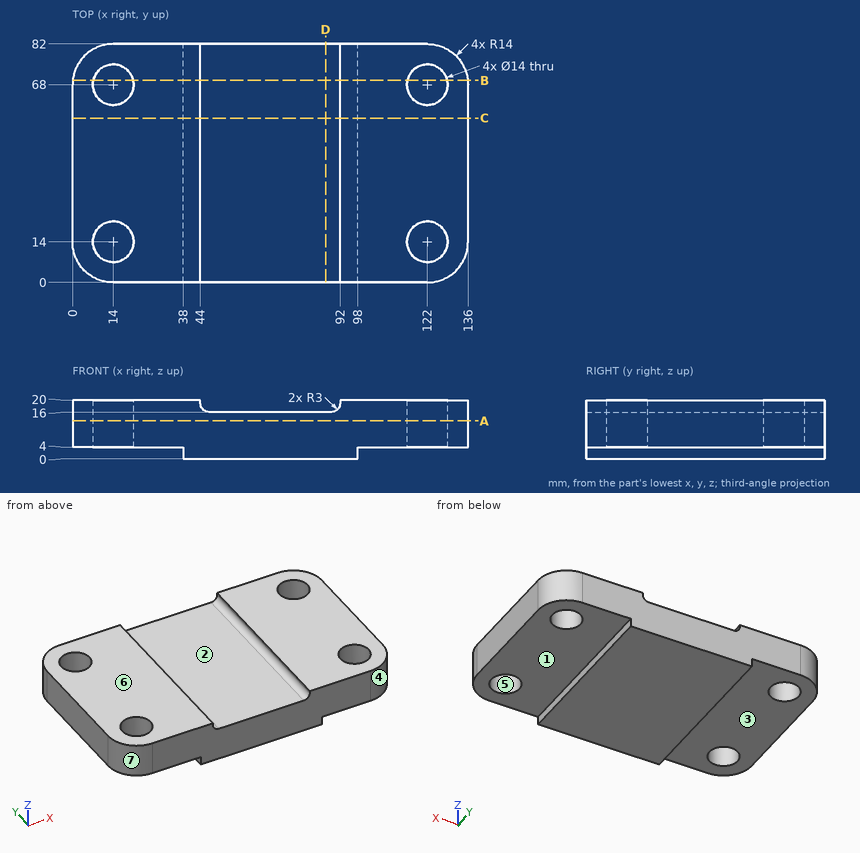
Drawing for the job (mm, zero at the part's lowest x, y, z). A direction names the side the tool comes from. Give positions to 0.01 mm unless a question says otherwise; leave off trailing zeros. Order: outer loops, then holes, each group sorted by start corner. A loop starts at its lowest first (then second) coordinate and runs counter-clockwise, first axis right, second up. Notation, with made-up numbers: M 36,-36 L 51,-36 A16 ccw 51,-9 Z; hole C -21.75,3.25 d11. An arc over 180 degrees is marked long. Write item = value, one per line. Start each with the question number.
(1) Which spindle directions (+Z, -Z, +X, -X, +Y, -Y) get a long thin tool onto all of the face, cutting with end or side? Do the marked faces 1, 2 and 3. Say none if no direction does.
(2) Slice it at A-A on z = 13. Write the cut outline in (x, y).
(3) Probe L1, parallel to Y at x = 14, z = 10.5; L2, parallel to X at y = 14.5, z = 16.5; L3, parallel to Y at x = 11, z = 12.5. List the from-to ranges inside material, lowest first. Write a range as [from, to].
(4) Two-plate mould, pull along X, no slides. Class the marked faces 4, 5, 6 and 7: released by +X, released by -X, zero draft, split by the parting line, or undercut.
(5) Slice it at D-D on x = 87. Write the cut outline in (y, z), plus the area to 3 significant figures.
(6) Slice it at B-B on y = 69.5. Write the cut outline in (x, z), plus the area to 3 significant figures.
(7) Pin check, flat tips, straight feed: pin 1 Ø11 at (x, y) = (122, 68) entering from +Z; pin 2 Ø2 at (x, y) = (109, 22) entering from -Z; pin 3 Ø5 at (x, y) = (85.5, 73) entering from +Z; pin 4 Ø4.5 at (y, z) = (56.5, 1) entering from -X. Stop position of each tip, or through.
(8) Slice it at C-C on y = 56.5. Write the cut outline in (x, z).
Responses:
q1.face_1 = -Z, +X, +Y, -Y
q1.face_2 = +Z, +Y, -Y
q1.face_3 = -Z, -X, +Y, -Y
q2.outline = M 0,14 A14 ccw 14,0 L 122,0 A14 ccw 136,14 L 136,68 A14 ccw 122,82 L 14,82 A14 ccw 0,68 Z; hole C 14,14 d14; hole C 14,68 d14; hole C 122,14 d14; hole C 122,68 d14
q3.L1 = [0, 7], [21, 61], [75, 82]
q3.L2 = [0, 7.02], [20.98, 45.34], [90.66, 115.02], [128.98, 136]
q3.L3 = [0.33, 7.68], [20.32, 61.68], [74.32, 81.67]
q4.face_4 = released by +X
q4.face_5 = undercut
q4.face_6 = zero draft
q4.face_7 = released by -X
q5.outline = M 0,0 L 82,0 L 82,16 L 0,16 Z
q5.area = 1,310 mm2
q6.outline = M 0.08,4 L 7.16,4 L 7.16,20 L 0.08,20 Z; M 20.84,4 L 38,4 L 38,0 L 98,0 L 98,4 L 115.16,4 L 115.16,20 L 92,20 L 92,19 A3 cw 89,16 L 47,16 A3 cw 44,19 L 44,20 L 20.84,20 Z; M 128.84,4 L 135.92,4 L 135.92,20 L 128.84,20 Z
q6.area = 1,790 mm2
q7.pin_1 = through
q7.pin_2 = 4
q7.pin_3 = 16
q7.pin_4 = 38
q8.outline = M 0,4 L 38,4 L 38,0 L 98,0 L 98,4 L 136,4 L 136,20 L 92,20 L 92,19 A3 cw 89,16 L 47,16 A3 cw 44,19 L 44,20 L 0,20 Z
